```python
from build123d import *

# Parameters (mm, degrees)
BOSS_EXTRUDE1_DEPTH = 152.4
CUT_EXTRUDE1_REACH  = 17.875
SKETCH3_R           = 1.6
CUT_EXTRUDE2_DEPTH  = 286.8
CUT_EXTRUDE3_REACH  = 17.875
SKETCH5_R           = 1.5875


with BuildPart() as part:
    # Sketch2 → Boss-Extrude1 (new body, symmetric)
    with BuildSketch(Plane.XY):
        with BuildLine():
            Line((-7.9375, 0), (7.9375, 0))
            Line((7.9375, 0), (7.9375, 15.875))
            Line((7.9375, 15.875), (7.14375, 15.875))
            ThreePointArc((7.14375, 15.875), (6.582483992, 15.642516008), (6.35, 15.08125))
            Line((6.35, 15.08125), (6.35, 2.38125))
            ThreePointArc((6.35, 2.38125), (6.117516008, 1.819983992), (5.55625, 1.5875))
            Line((5.55625, 1.5875), (-7.14375, 1.5875))
            ThreePointArc((-7.14375, 1.5875), (-7.705016008, 1.355016008), (-7.9375, 0.79375))
            Line((-7.9375, 0.79375), (-7.9375, 0))
        make_face()
    extrude(amount=BOSS_EXTRUDE1_DEPTH, both=True)

    # Sketch3 → Cut-Extrude1 (cut, up to next)
    with BuildSketch(Plane(origin=(7.9375, 0, 0), x_dir=(0, 0, -1), z_dir=(1, 0, 0)), mode=Mode.PRIVATE) as cut_extrude1_sk1:
        with Locations((148.4, 7.9375)):
            Circle(SKETCH3_R)
    cut_extrude1_tool1 = extrude(cut_extrude1_sk1.sketch, amount=-CUT_EXTRUDE1_REACH, mode=Mode.PRIVATE) & part.part
    add(cut_extrude1_tool1.solids().sort_by_distance((7.9375, 7.9375, -148.4))[0], mode=Mode.SUBTRACT)
    # Sketch3 → Cut-Extrude1 (cut, up to next)
    with BuildSketch(Plane(origin=(7.9375, 0, 0), x_dir=(0, 0, -1), z_dir=(1, 0, 0)), mode=Mode.PRIVATE) as cut_extrude1_sk2:
        with Locations((140.4, 7.9375)):
            Circle(SKETCH3_R)
    cut_extrude1_tool2 = extrude(cut_extrude1_sk2.sketch, amount=-CUT_EXTRUDE1_REACH, mode=Mode.PRIVATE) & part.part
    add(cut_extrude1_tool2.solids().sort_by_distance((7.9375, 7.9375, -140.4))[0], mode=Mode.SUBTRACT)

    # Sketch4 → Cut-Extrude2 (cut)
    with BuildSketch(Plane.XY.offset(152.4)):
        with BuildLine():
            Line((-7.9375, 0.79375), (-7.9375, 0))
            Line((-7.9375, 0), (7.9375, 0))
            Line((7.9375, 0), (7.9375, 15.875))
            Line((7.9375, 15.875), (7.14375, 15.875))
            ThreePointArc((7.14375, 15.875), (6.582483992, 15.642516008), (6.35, 15.08125))
            Line((6.35, 15.08125), (6.35, 2.38125))
            ThreePointArc((6.35, 2.38125), (6.117516008, 1.819983992), (5.55625, 1.5875))
            Line((5.55625, 1.5875), (-7.14375, 1.5875))
            ThreePointArc((-7.14375, 1.5875), (-7.705016008, 1.355016008), (-7.9375, 0.79375))
        make_face()
    extrude(amount=-CUT_EXTRUDE2_DEPTH, mode=Mode.SUBTRACT)

    # Sketch5 → Cut-Extrude3 (cut, up to next)
    with BuildSketch(Plane.XZ, mode=Mode.PRIVATE) as cut_extrude3_sk1:
        with Locations((0, -143.4)):
            Circle(SKETCH5_R)
    cut_extrude3_tool1 = extrude(cut_extrude3_sk1.sketch, amount=-CUT_EXTRUDE3_REACH, mode=Mode.PRIVATE) & part.part
    add(cut_extrude3_tool1.solids().sort_by_distance((0, 0, -143.4))[0], mode=Mode.SUBTRACT)


solid = part.part
```
Can you work these out from the model? Positions are in its coordinate system, mm. A direction names the side the tool comes from. Give positions to 0.01 mm unless a question says otherwise; leave off trailing zeros. Write each loop counter-clockwise with the first axis right and the second up, starting at its lowest first coordinate (ties: lowest second). Pieces come first, ordered by that corner, then holes. Notation, with made-up numbers: (-18.75, 47.25) -> (-10.75, 47.25) arc R7 cw to (-10.75, 54.25) -> close; hole circle Ø5 at (0, -12.5). An arc over 180 degrees is marked (long way). One line per item, written item: value.
Q1. Which directions (+Z, -Z, +X, -X, +Y, -Y) give clear straight access to the entire face, cutting with the end or side of a thin tool? Please do faces 4 (the face through (7.938, 8, -143)), 5 (the face through (-2, 1.588, -143)).
Results found:
face 4: +Z, -Z, +X, +Y, -Y
face 5: +Z, -Z, -X, +Y
Q2. We'd pull the mould along Y, two halves only. Please class faces 1 (the face through (-0.207, 0.783, -141.826)), 2 (the face through (2, 0, -143)), 3 (the face through (7.155, 7.325, -149.878)): +Y half, -Y half, draft (parallel to the pull), parting line (faces both ways), or undercut.
Results found:
face 1: draft
face 2: -Y half
face 3: undercut
Q3. Imagine slicing it at B-B on x = -0.5. Please give me the cut outline in (y, z).
Results found:
outline: (0, -152.4) -> (1.59, -152.4) -> (1.59, -144.91) -> (0, -144.91) -> close; (0, -141.89) -> (1.59, -141.89) -> (1.59, -134.4) -> (0, -134.4) -> close
Q4. Please list where these lines run through material, in increasing order: line 1 (Y direction, x = 7.25, z = -148.4) (1 decimal); line 2 (Z direction, x = 0, y = 0.5); line 3 (Y direction, x = -3, z = -137). Write a range as [from, to].
Results found:
line 1: y = [0, 6.3], [9.5, 15.9]
line 2: z = [-152.4, -144.99], [-141.81, -134.4]
line 3: y = [0, 1.59]
Q5. For P1, Ø2, axis at x = -3, z = -144, coming from the +Y side; P2, Ø4, axis at y = 7.94, z = -148.4, coming from the -X side, each with a flat end and sliding along its axis, tell me the tip position at first contact or that it passes through.
Results found:
P1: stops at y = 1.59
P2: stops at x = 6.35
Q6. Imagine slicing it at D-D on x = 4. Please give me the cut outline in (y, z).
Results found:
outline: (0, -152.4) -> (1.59, -152.4) -> (1.59, -134.4) -> (0, -134.4) -> close
